```python
from build123d import *

# Parameters (mm, degrees)
SKETCH1_R                 = 14.29004
BOSS_EXTRUDE1_DEPTH       = 4.7625
F_10_CLEARANCE_HOLE1_D    = 4.9784
F_10_CLEARANCE_HOLE2_D    = 4.9784
TAP_DRILL_FOR_8_32_TAP1_D = 3.4544
F_10_CLEARANCE_HOLE3_D    = 4.9784
FILLET1_R                 = 1.5875


with BuildPart() as part:
    # Sketch1 → Boss-Extrude1 (new body)
    with BuildSketch(Plane(origin=(0, 0, 0), x_dir=(1, 0, 0), z_dir=(0, 1, 0))):
        with BuildLine():
            Line((-62.038222018, -79.883349745), (25.167081601, -41.695780276))
            ThreePointArc((25.167081601, -41.695780276), (34.91524479, -34.148496119), (39.940188099, -22.890693115))
            Line((39.940188099, -22.890693115), (42.275148896, -9.586739751))
            Line((42.275148896, -9.586739751), (65.831008632, 16.012754812))
            Line((65.831008632, 16.012754812), (65.831008632, 61.493591694))
            Line((65.831008632, 61.493591694), (28.046575186, 61.493591694))
            ThreePointArc((28.046575186, 61.493591694), (13.665119108, 55.581463016), (7.599980341, 41.263864189))
            Line((7.599980341, 41.263864189), (7.377499016, 31.276274442))
            ThreePointArc((7.377499016, 31.276274442), (0.022382465, 13.519452313), (-17.734439664, 6.164335762))
            Line((-17.734439664, 6.164335762), (-92.776174625, 6.164335762))
            Line((-92.776174625, 6.164335762), (-106.671272051, 28.401139958))
            Line((-106.671272051, 28.401139958), (-135.754553791, 28.401139958))
            Line((-135.754553791, 28.401139958), (-135.754553791, 20.45773786))
            Line((-135.754553791, 20.45773786), (-138.929553791, 17.28273786))
            Line((-138.929553791, 17.28273786), (-138.929553791, 6.164335762))
            Line((-138.929553791, 6.164335762), (-135.754553791, 6.164335762))
            Line((-135.754553791, 6.164335762), (-135.754553791, -3.360664238))
            Line((-135.754553791, -3.360664238), (-124.263208355, -3.360664238))
            Line((-124.263208355, -3.360664238), (-110.958501432, -24.652646126))
            Line((-110.958501432, -24.652646126), (-107.963388287, -24.652646126))
            Line((-107.963388287, -24.652646126), (-97.659911134, -41.141656383))
            Line((-97.659911134, -41.141656383), (-97.659911134, -56.628468385))
            ThreePointArc((-97.659911134, -56.628468385), (-86.144175153, -77.898718987), (-62.038222018, -79.883349745))
        make_face()
        with Locations(Location((28.046575186, 41.045834415, 0), (0, 0, 90))):
            Circle(SKETCH1_R, mode=Mode.SUBTRACT)
        with Locations(Location((15.031008632, -18.508482198, 0), (0, 0, 90))):
            Circle(SKETCH1_R, mode=Mode.SUBTRACT)
        with Locations(Location((-72.258332946, -56.628468385, 0), (0, 0, 90))):
            Circle(SKETCH1_R, mode=Mode.SUBTRACT)
    extrude(amount=BOSS_EXTRUDE1_DEPTH)

    # #10 Clearance Hole1 (through all)
    with Locations(Plane(origin=(0, 4.7625, 0), x_dir=(1, 0, 0), z_dir=(0, 1, 0))):
        with Locations((61.830508632, 55.024283038), (61.830508632, 27.084283038), (-130.992053791, 23.944335762), (-130.992053791, 1.084335762)):
            Hole(F_10_CLEARANCE_HOLE1_D / 2)

    # #10 Clearance Hole2 (through all)
    with Locations(Plane(origin=(0, 4.7625, 0), x_dir=(1, 0, 0), z_dir=(0, 1, 0))):
        with Locations((-110.620877013, -13.210000682), (-94.465560781, -3.115038698), (-112.732400526, 8.143579493)):
            Hole(F_10_CLEARANCE_HOLE2_D / 2)

    # Tap Drill for #8-32 Tap1 (through all)
    with Locations(Plane(origin=(0, 4.7625, 0), x_dir=(1, 0, 0), z_dir=(0, 1, 0))):
        with Locations((-85.010296638, -43.876504694), (-59.506369254, -69.380432077), (2.27904494, -31.26044589), (27.782972324, -5.756518506), (15.294611495, 28.293870723), (40.798538878, 53.797798107)):
            Hole(TAP_DRILL_FOR_8_32_TAP1_D / 2)

    # #10 Clearance Hole3 (through all)
    with Locations(Plane(origin=(0, 4.7625, 0), x_dir=(1, 0, 0), z_dir=(0, 1, 0))):
        with Locations((-56.041369259, -27.019222928), (-8.951277081, -51.090630662)):
            Hole(F_10_CLEARANCE_HOLE3_D / 2)

    # Fillet1
    fillet1_edges = [part.edges().sort_by_distance(p)[0] for p in [
        (-135.754553791, 2.38125, -20.45773786),
        (-135.754553791, 2.38125, -28.401139958),
        (-106.671272051, 2.38125, -28.401139958),
        (-92.776174625, 2.38125, -6.164335762),
        (65.831008632, 2.38125, -61.493591694),
        (65.831008632, 2.38125, -16.012754812),
        (42.275148896, 2.38125, 9.586739751),
        (-97.659911134, 2.38125, 41.141656383),
        (-107.963388287, 2.38125, 24.652646126),
        (-110.958501432, 2.38125, 24.652646126),
        (-124.263208355, 2.38125, 3.360664238),
        (-135.754553791, 2.38125, 3.360664238),
        (-138.929553791, 2.38125, -6.164335762),
        (-138.929553791, 2.38125, -17.28273786),
    ]]
    fillet(fillet1_edges, radius=FILLET1_R)


solid = part.part
```
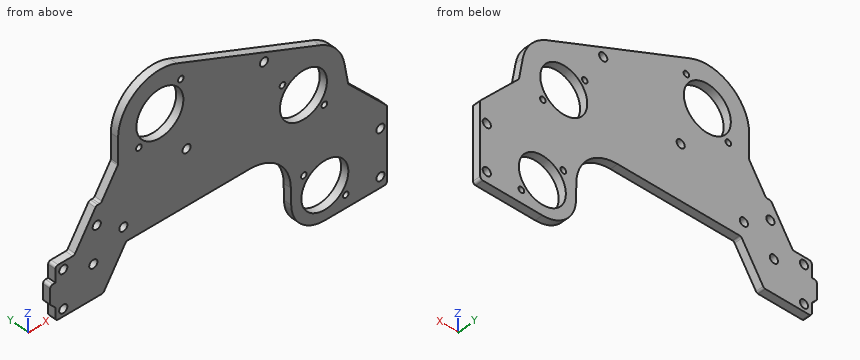
Work out the finished part from the listing and answer in its coordinate system (mm). Coordinates: 2 decimals unless noted, no trailing zeros. Loops run counter-clockwise (first coordinate to the right, second up) from the corner with the lowest first, then second, coordinate; pieces in that order, holes last. Notation, with made-up numbers: M -4.5,15.25 L 2.5,15.25 A19 cw 2.5,39.25 Z; hole C -12.5,-6.5 d11. An arc over 180 degrees is marked long. Use CSV: the item, a comma, the result in double quotes. Start each with the question number.
(1) Find section C-C, the plane z = 13.21. Give the vertices of the cut face in (x, y), then the cut area to 3 significant figures.
(2) Find section D-D, the plane y = 1.5. State how many separate pieces and enclosed holes the cut face has, then the cut area to 3 significant figures.
(3) Consider line 1 (Z direction, x = -130.5, y = 4.05); line 2 (X direction, y = 1.9, z = 25.5); line 3 (X direction, y = 0.8, z = -25). Determine where each line is inside the solid, lowest interval first.
(4) Find section A-A, the plane x = -9. Give the vertices of the cut face in (y, z), then the cut area to 3 significant figures.
(5) Find section B-B, the plane z = 59.5. Give the vertices of the cut face in (x, y), then the cut area to 3 significant figures.
(6) Given pin 1 Ø1.5 at (y, z) = (4, 60) entering from -X; pin 2 Ø17 at (x, z) = (-72.26, 56.63) entering from +Y; pin 3 Ø1.4 at (y, z) = (1.5, 48.5) entering from -X, each flat-ended and moving along its own axis, determine where each tip first touches the part or whether it passes through.
Recorded:
1,outline,"M -118.11,0 L -113.11,0 L -113.11,4.76 L -118.11,4.76 Z; M -108.13,0 L 1.76,0 L 1.76,4.76 L -108.13,4.76 Z; M 28.3,0 L 41.64,0 L 41.64,4.76 L 28.3,4.76 Z"
1,area,"611 mm^2"
2,separate pieces,"1"
2,enclosed holes,"18"
2,area,"12,400 mm^2"
3,line 1,"z = -28.4 to -26.38, -21.5 to -3.52, 1.36 to 3.36"
3,line 2,"x = -107.43 to -58.01, -54.07 to 2.57, 27.49 to 39.34"
3,line 3,"x = -135.75 to -133.25, -128.74 to -104.55, 6.58 to 60.47, 63.19 to 65.83"
4,outline,"M 0,-7.73 L 4.76,-7.73 L 4.76,48.6 L 0,48.6 Z; M 0,53.58 L 4.76,53.58 L 4.76,56.66 L 0,56.66 Z"
4,area,"283 mm^2"
5,outline,"M -97.5,0 L -86.26,0 L -86.26,4.76 L -97.5,4.76 Z; M -58.26,0 L -15.49,0 L -15.49,4.76 L -58.26,4.76 Z"
5,area,"257 mm^2"
6,pin 1,"stops at x = -97.52"
6,pin 2,"passes through"
6,pin 3,"stops at x = -97.66"
